from build123d import *

# Parameters (mm, degrees)
F0_W         = 116
F0_H         = 24
F1_DEPTH     = 3
F2_R         = 2
F3_T1_DEPTH  = 6
F3_S5_W      = 2
F3_S5_H      = 2
F3_T6_DEPTH  = 2
F3_S11_W     = 2
F3_S11_H     = 2
F3_T12_DEPTH = 2
F3_S17_W     = 2
F3_S17_H     = 2
F3_T18_DEPTH = 2
F3_S23_W     = 2
F3_S23_H     = 2
F3_T24_DEPTH = 2


# Not quite as in the source:
# - a fillet or chamfer that OpenCascade refuses, or shapes differently, is made with other operations: its cross-section is extruded or revolved along the edge and cut away or added


with BuildPart() as f1:
    # F0 (on Top) → F1 (new body)
    with BuildSketch(Plane.XY):
        Rectangle(F0_W, F0_H)
    extrude(amount=F1_DEPTH)

    # F2
    f2_edges = [f1.edges().sort_by_distance(p)[0] for p in [
        (58, 0, 3),
        (0, 12, 3),
        (-58, 0, 3),
        (0, -12, 3),
    ]]
    fillet(f2_edges, radius=F2_R)

    # F3: fillet of radius 2 on 4 edges, made by hand

    # F3_s2 → F3_t1 (cut)
    with BuildSketch(Plane.XY.offset(-5)):
        with BuildLine():
            ThreePointArc((58, -10), (57.4142135624, -11.4142135624), (56, -12))
            Line((56, -12), (58, -12))
            Line((58, -12), (58, -10))
        make_face()
        with BuildLine():
            ThreePointArc((58, 10), (57.4142135624, 11.4142135624), (56, 12))
            Line((56, 12), (58, 12))
            Line((58, 12), (58, 10))
        make_face()
        with BuildLine():
            ThreePointArc((-56, -12), (-57.4142135624, -11.4142135624), (-58, -10))
            Line((-58, -10), (-58, -12))
            Line((-58, -12), (-56, -12))
        make_face()
        with BuildLine():
            ThreePointArc((-56, 12), (-57.4142135624, 11.4142135624), (-58, 10))
            Line((-58, 10), (-58, 12))
            Line((-58, 12), (-56, 12))
        make_face()
    extrude(amount=F3_T1_DEPTH, mode=Mode.SUBTRACT)


with BuildPart() as f3_tool4:
    # F3_s5 → F3_t6 (new body)
    with BuildSketch(Plane.XZ.offset(-10)):
        with Locations((-57, 2)):
            Rectangle(F3_S5_W, F3_S5_H)
    extrude(amount=-F3_T6_DEPTH)

    # F3_s7 → F3_t8 (revolve, cut)
    with BuildSketch(Plane(origin=(-56, 10, 1), x_dir=(0.7071067812, 0, -0.7071067812), z_dir=(0.7071067812, 0, 0.7071067812))):
        with BuildLine():
            ThreePointArc((0, -2), (2, 0), (0, 2))
            Line((0, 2), (0, -2))
        make_face()
    revolve(axis=Axis((-56, 10, 1), (0, 1, 0)), mode=Mode.SUBTRACT)


with BuildPart() as f1_1:
    add(f1.part)

    # F3_t3: cut F3_tool4
    add(f3_tool4.part, mode=Mode.SUBTRACT)


with BuildPart() as f3_tool10:
    # F3_s11 → F3_t12 (new body)
    with BuildSketch(Plane.XZ.offset(10)):
        with Locations((-57, 2)):
            Rectangle(F3_S11_W, F3_S11_H)
    extrude(amount=F3_T12_DEPTH)

    # F3_s13 → F3_t14 (revolve, cut)
    with BuildSketch(Plane(origin=(-56, -10, 1), x_dir=(0.7071067812, 0, -0.7071067812), z_dir=(-0.7071067812, 0, -0.7071067812))):
        with BuildLine():
            ThreePointArc((0, -2), (2, 0), (0, 2))
            Line((0, 2), (0, -2))
        make_face()
    revolve(axis=Axis((-56, -10, 1), (0, -1, 0)), mode=Mode.SUBTRACT)


with BuildPart() as f1_2:
    add(f1_1.part)

    # F3_t9: cut F3_tool10
    add(f3_tool10.part, mode=Mode.SUBTRACT)


with BuildPart() as f3_tool16:
    # F3_s17 → F3_t18 (new body)
    with BuildSketch(Plane.YZ.offset(56)):
        with Locations((11, 2)):
            Rectangle(F3_S17_W, F3_S17_H)
    extrude(amount=F3_T18_DEPTH)

    # F3_s19 → F3_t20 (revolve, cut)
    with BuildSketch(Plane(origin=(56, 10, 1), x_dir=(0, -0.7071067812, -0.7071067812), z_dir=(0, -0.7071067812, 0.7071067812))):
        with BuildLine():
            ThreePointArc((0, -2), (2, 0), (0, 2))
            Line((0, 2), (0, -2))
        make_face()
    revolve(axis=Axis((56, 10, 1), (1, 0, 0)), mode=Mode.SUBTRACT)


with BuildPart() as f1_3:
    add(f1_2.part)

    # F3_t15: cut F3_tool16
    add(f3_tool16.part, mode=Mode.SUBTRACT)


with BuildPart() as f3_tool22:
    # F3_s23 → F3_t24 (new body)
    with BuildSketch(Plane.YZ.offset(56)):
        with Locations((-11, 2)):
            Rectangle(F3_S23_W, F3_S23_H)
    extrude(amount=F3_T24_DEPTH)

    # F3_s25 → F3_t26 (revolve, cut)
    with BuildSketch(Plane(origin=(56, -10, 1), x_dir=(0, 0.7071067812, -0.7071067812), z_dir=(0, -0.7071067812, -0.7071067812))):
        with BuildLine():
            ThreePointArc((0, -2), (2, 0), (0, 2))
            Line((0, 2), (0, -2))
        make_face()
    revolve(axis=Axis((56, -10, 1), (1, 0, 0)), mode=Mode.SUBTRACT)


with BuildPart() as f1_4:
    add(f1_3.part)

    # F3_t21: cut F3_tool22
    add(f3_tool22.part, mode=Mode.SUBTRACT)


solid = f1_4.part
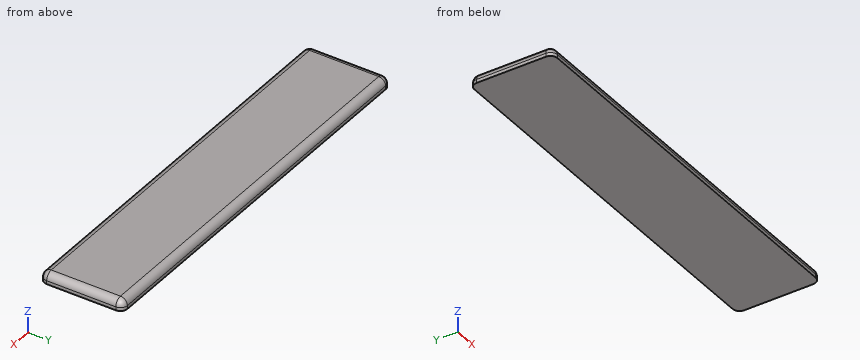
For this review, take the finished solid that the model builds, in its own axes (mm). Round coordinates to 2 decimals unless told otherwise and drop trailing zeros. Write each loop counter-clockwise with the first axis right and the second up, starting at its lowest first coordinate (ties: lowest second). Pieces come first, ordered by that corner, then holes. Notation, with made-up numbers: (27.25, 1) -> (59.25, 1) arc R9 cw to (59.25, 14) -> close; hole circle Ø5 at (31.25, 84.5). An arc over 180 degrees is marked (long way). Use CSV: the item, a comma, the result in double quotes.
(1) Consider section A-A, the plane x = 10. Give the boundary of the cut face in (y, z).
Computed values:
outline,"(-12, 0) -> (12, 0) -> (12, 1) arc R2 ccw to (10, 3) -> (-10, 3) arc R2 ccw to (-12, 1) -> close"
(2) Clearance check with a flat-ended pin moving along its axis: P1, Ø1.5, axis at x = 28.5, y = -4.5, coming from the -Z side. State where the tip first meets the part, or that it passes through.
Computed values:
P1,"z = 0"
(3) To check wall thickness, follow L1, parallel to Y at x = -5.5, z = 1.3; L2, parallel to Z at x = -9.5, y = 10.75; L3, parallel to Y at x = -44.5, z = 1.65. State the ranges of each line that lie inside material, in increasing order. Write a range as [from, to].
Computed values:
L1,"[-11.98, 11.98]"
L2,"[0, 2.85]"
L3,"[-11.89, 11.89]"
